Verification items for the finished model (mm, model axes). Give positions to 0.01 mm unless a question says otherwise; leave off trailing zeros. Answer as a JSON object with one key per item and string values. Group by question number.
Item 1: Scan lines: line 1 along X through (y, z) = (-139.7, -5); line 2 along Z through (x, y) = (21.75, -38.1). Record each from-to range of solid material in increasing order. Write a range as [from, to].
Item 2: Sectioned sample at A-A, the plane z = -4.25. Count the separate pieces of the cut face and the enclosed holes in it, and give its area (3 significant figures).
Item 3: Go/stop test with flat-tipped pins: pin 1 (6.5 mm diameter, centred on y = -63.5, z = -12.7, fed in from -X); pin 2 (3.5 mm diameter, centred on y = -139.7, z = -12.7, fed in from -X). Record where each tip stops, or that it passes through.
Autodesk Inventor part; units mm, degrees
ref_plane "YZ Plane" through (0, 0, 0) normal (1, 0, 0) x (0, 1, 0)
ref_plane "XZ Plane" through (0, 0, 0) normal (0, 1, 0) x (-1, 0, 0)
ref_plane "XY Plane" through (0, 0, 0) normal (0, 0, 1) x (1, 0, 0)
sketch "Sketch1" plane through (0, 0, 0) normal (0, 0, 1) x (1, 0, 0)
  line L0 (0, 0) -> (25.4, 0)
  line L1 (25.4, 0) -> (25.4, -304.8)
  line L2 (25.4, -304.8) -> (0, -304.8)
  line L3 (0, -304.8) -> (0, 0)
  dimension "d0" = 304.8
  dimension "d1" = 25.4
extrude "Extrusion1" add sketch "Sketch1" against normal blind 25.4
sketch "Sketch2" plane through (0, 0, 0) normal (0, 0, 1) x (1, 0, 0)
  circle A0 centre (12.7, -12.7) radius 1.9685
  line L0 (25.4, 0) -> (25.4, -304.8)
  line L1 (0, 0) -> (25.4, 0)
  circle A1 centre (12.7, -38.1) radius 1.9685
  circle A2 centre (12.7, -63.5) radius 1.9685
  circle A3 centre (12.7, -88.9) radius 1.9685
  circle A4 centre (12.7, -114.3) radius 1.9685
  circle A5 centre (12.7, -139.7) radius 1.9685
  circle A6 centre (12.7, -165.1) radius 1.9685
  circle A7 centre (12.7, -190.5) radius 1.9685
  circle A8 centre (12.7, -215.9) radius 1.9685
  circle A9 centre (12.7, -241.3) radius 1.9685
  circle A10 centre (12.7, -266.7) radius 1.9685
  circle A11 centre (12.7, -292.1) radius 1.9685
  dimension "d5" = 3.937
  dimension "d6" = 12.7
  dimension "d7" = 12.7
  dimension "d10" = 25.4
extrude "Extrusion2" cut sketch "Sketch2" against normal blind 304.8
sketch "Sketch3" plane through (25.4, -304.8, 0) normal (1, 0, 0) x (0, 0, -1)
  circle A0 centre (12.7, 292.1) radius 1.9685
  line L0 (0, 304.8) -> (25.4, 304.8)
  line L1 (25.4, 304.8) -> (25.4, 0)
  circle A1 centre (12.7, 266.7) radius 1.9685
  circle A2 centre (12.7, 241.3) radius 1.9685
  circle A3 centre (12.7, 215.9) radius 1.9685
  circle A4 centre (12.7, 190.5) radius 1.9685
  circle A5 centre (12.7, 165.1) radius 1.9685
  circle A6 centre (12.7, 139.7) radius 1.9685
  circle A7 centre (12.7, 114.3) radius 1.9685
  circle A8 centre (12.7, 88.9) radius 1.9685
  circle A9 centre (12.7, 63.5) radius 1.9685
  circle A10 centre (12.7, 38.1) radius 1.9685
  circle A11 centre (12.7, 12.7) radius 1.9685
  dimension "d17" = 3.937
  dimension "d18" = 12.7
  dimension "d19" = 12.7
  dimension "d22" = 25.4
extrude "Extrusion3" cut sketch "Sketch3" against normal blind 304.8
properties part number "Frame 10"
Geometry check:
{
 "1": {"line 1": "[0, 10.73], [14.67, 25.4]", "line 2": "[-25.4, -14.67], [-10.73, 0]"},
 "2": {"separate pieces": "1", "enclosed holes": "12", "area": "7,600 mm^2"},
 "3": {"pin 1": "x = 0", "pin 2": "through"}
}
